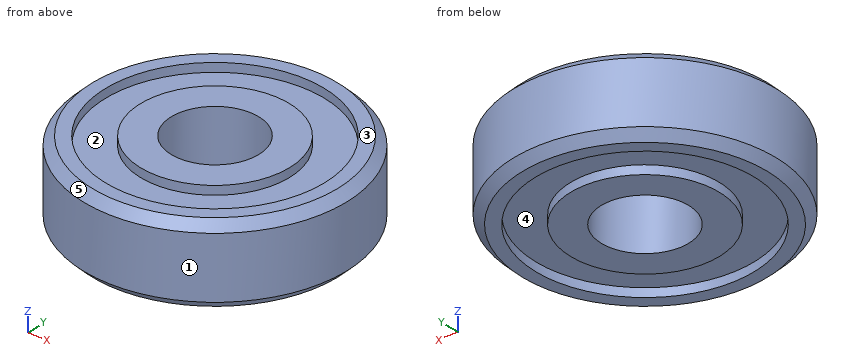
```python
from build123d import *

# Parameters (mm, degrees)
SKETCH_R      = 8.5
SKETCH_R_2    = 5
PAD_DEPTH     = 9
SKETCH001_R   = 12.5
SKETCH001_R_2 = 8.5
PAD001_DEPTH  = 7
SKETCH002_R   = 15
SKETCH002_R_2 = 12.5
PAD002_DEPTH  = 9
CHAMFER_SIZE  = 1


with BuildPart() as part:
    # Sketch → Pad (new body)
    with BuildSketch(Plane.XY):
        Circle(SKETCH_R)
        Circle(SKETCH_R_2, mode=Mode.SUBTRACT)
    extrude(amount=PAD_DEPTH)

    # Sketch001 (on Face3 of Pad) → Pad001 (join)
    with BuildSketch(Plane(origin=(0, 0, 1), x_dir=(1, 0, 0), z_dir=(0, 0, -1))):
        Circle(SKETCH001_R)
        Circle(SKETCH001_R_2, mode=Mode.SUBTRACT)
    extrude(amount=-PAD001_DEPTH)

    # Sketch002 (on Face2 of Pad001) → Pad002 (join)
    with BuildSketch(Plane(origin=(0, 0, 0), x_dir=(1, 0, 0), z_dir=(0, 0, -1))):
        Circle(SKETCH002_R)
        Circle(SKETCH002_R_2, mode=Mode.SUBTRACT)
    extrude(amount=-PAD002_DEPTH)

    # Chamfer
    chamfer_edges = [part.edges().sort_by_distance(p)[0] for p in [
        (-15, 0, 9),
        (-15, 0, 0),
    ]]
    chamfer(chamfer_edges, length=CHAMFER_SIZE)


solid = part.part
```
Geometry check sheet. Reference: the model listing, model coordinates, mm. Face numbers are marked on the shaded views. A direction names the side the tool comes from. Round coordinates to 2 decimals unless told otherwise and drop trailing zeros. Order: outer loops, then holes, each group sorted by start corner. A loop starts at its lowest first (then second) coordinate and runs counter-clockwise, first axis right, second up. Notation, with made-up numbers: M 75,-20 L 115,-20 A18 cw 115,3 Z; hole C -32.75,0.5 d4. An arc over 180 degrees is marked long. Answer as CSV lines item,"result".
1) Tool access check on the marked faces 1 and 2. Record the directions out of +Z, -Z, +X, -X, +Y, -Y that give a thin tool (end or side, any length) a straight path to the whole face; none if there is none.
Entries:
face 1,"+Z, -Z"
face 2,"+Z"
2) Thickness scan on probe 1 along Y at (x, z) = (0, 8.55); probe 2 along Y at (x, z) = (0, 0.7); probe 3 along Z at (x, y) = (11, 4). Record the ranges inside material, lowest first. Write a range as [from, to].
Entries:
probe 1,"[-14.45, -12.5], [-8.5, -5], [5, 8.5], [12.5, 14.45]"
probe 2,"[-14.7, -12.5], [-8.5, -5], [5, 8.5], [12.5, 14.7]"
probe 3,"[1, 8]"
3) Gauge pin test, flat ends, axial feed: pin 1 Ø3 at (y, z) = (-8, 6) entering from +X; pin 2 Ø6 at (x, y) = (0, 0) entering from +Z. Record the tip position at first contact, or that the pin passes through.
Entries:
pin 1,"x = 13.52"
pin 2,"through"
4) Sectioned sample at A-A on y = 0. Record the cut outline in (x, z), and give its area (3 significant figures).
Entries:
outline,"M -15,1 L -14,0 L -12.5,0 L -12.5,1 L -8.5,1 L -8.5,0 L -5,0 L -5,9 L -8.5,9 L -8.5,8 L -12.5,8 L -12.5,9 L -14,9 L -15,8 Z; M 5,0 L 8.5,0 L 8.5,1 L 12.5,1 L 12.5,0 L 14,0 L 15,1 L 15,8 L 14,9 L 12.5,9 L 12.5,8 L 8.5,8 L 8.5,9 L 5,9 Z"
area,"162 mm2"
5) Sectioned sample at C-C on z = 0.5. Record the cut outline in (x, y).
Entries:
outline,"C 0,0 d29; C 0,0 d17; hole C 0,0 d25; hole C 0,0 d10"
6) Mould release check, pull along X, two halves, no side actions. Record for the marked faces 3, 4 and 5: +X half, -X half, draft (parallel to the pull), parting line (faces both ways), or undercut.
Entries:
face 3,"draft"
face 4,"undercut"
face 5,"parting line"
7) Sectioned sample at D-D on z = 7. Record the cut outline in (x, y).
Entries:
outline,"C 0,0 d30; hole C 0,0 d10"
